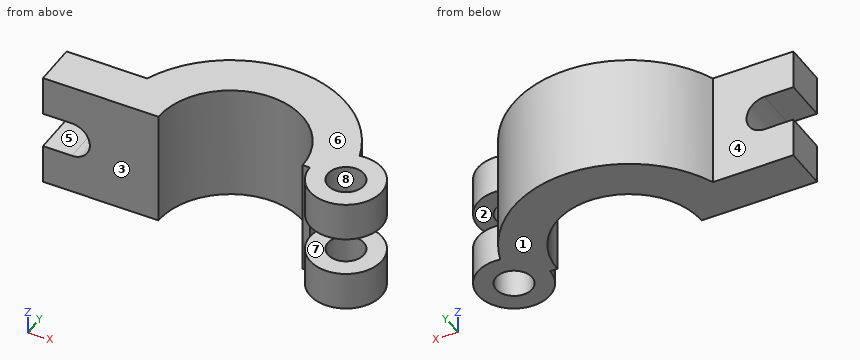
```python
from build123d import *

# Parameters (mm, degrees)
BOSS_EXTRUDE1_DEPTH     = 4
SKETCH2_R               = 2.5
BOSS_EXTRUDE3_DEPTH     = 4
SKETCH3_R               = 1.25
CUT_EXTRUDE1_DEPTH      = 8
SKETCH4_R               = 2.5
CUT_EXTRUDE2_DEPTH      = 1.333333333
CUT_EXTRUDE3_DEPTH      = 15.671400751
CUT_EXTRUDE3_DEPTH_BACK = 3


with BuildPart() as part:
    # Sketch1 → Boss-Extrude1 (new, symmetric)
    with BuildSketch(Plane.XY):
        with BuildLine():
            ThreePointArc((-8, 0), (0, 8), (8, 0))
            Line((8, 0), (5, 0))
            ThreePointArc((5, 0), (0, 5), (-5, 0))
            Line((-5, 0), (-8, 0))
        make_face()
        with BuildLine():
            Line((-13, 0), (-8, 0))
            ThreePointArc((-8, 0), (-7.85269342, 1.5281381), (-7.416198487, 3))
            Line((-7.416198487, 3), (-13, 3))
            Line((-13, 3), (-13, 0))
        make_face()
    extrude(amount=BOSS_EXTRUDE1_DEPTH, both=True)

    # Sketch2 → Boss-Extrude3 (add, symmetric)
    with BuildSketch(Plane.XY):
        with Locations((8, 0)):
            Circle(SKETCH2_R)
    extrude(amount=BOSS_EXTRUDE3_DEPTH, both=True)

    # Sketch3 → Cut-Extrude1 (cut)
    with BuildSketch(Plane.XY.offset(4)):
        with Locations((8, 0)):
            Circle(SKETCH3_R)
    extrude(amount=-CUT_EXTRUDE1_DEPTH, mode=Mode.SUBTRACT)

    # Sketch4 → Cut-Extrude2 (cut, symmetric)
    with BuildSketch(Plane.XY):
        with Locations((8, 0)):
            Circle(SKETCH4_R)
    extrude(amount=CUT_EXTRUDE2_DEPTH, both=True, mode=Mode.SUBTRACT)

    # Sketch5 → Cut-Extrude3 (cut, two sides: drawn at the far end of the back side and taken through both)
    with BuildSketch(Plane(origin=(0, 3, 0), x_dir=(1, 0, 0), z_dir=(0, 1, 0)).offset(-CUT_EXTRUDE3_DEPTH_BACK)):
        with BuildLine():
            Line((-11, 1.25), (-13, 1.25))
            Line((-13, 1.25), (-13, -1.25))
            Line((-13, -1.25), (-11, -1.25))
            ThreePointArc((-11, -1.25), (-9.75, 0), (-11, 1.25))
        make_face()
    extrude(amount=CUT_EXTRUDE3_DEPTH + CUT_EXTRUDE3_DEPTH_BACK, mode=Mode.SUBTRACT)


solid = part.part
```
Part model, mm, in its own coordinate system. Face numbers are marked on the shaded views. A direction names the side the tool comes from. Coordinates: 2 decimals unless noted, no trailing zeros. Order: outer loops, then holes, each group sorted by start corner. A loop starts at its lowest first (then second) coordinate and runs counter-clockwise, first axis right, second up. Notation, with made-up numbers: (-15.75, -8.5) -> (12.25, -8.5) arc R30 cw to (12.25, 26.5) -> close; hole circle Ø1 at (78, -20). An arc over 180 degrees is marked (long way). Put each result on its own line as item: value. Start each with the question number.
(1) Band-saw the part on A-A (z = 3.25). Give the cut face in (x, y).
(2) Band-saw the part on B-B (x = 8). Give the cut face in (y, z).
(3) Band-saw the part on C-C (y = 4.25). Give the cut face in (x, z).
(4) Band-saw the part on D-D (y = 0.5). Give the cut face in (x, z).
(5) Mould opens along Z. For the marked faces 6, 7 and 8 say: pulls with the +Z half, pulls with the -Z half, needs draft (parallel to the pull), parting line crosses it, or undercut.
(6) Pin check, flat tips, straight feed: pin 1 Ø2.5 at (x, y) = (9, 0.5) entering from -Z; pin 2 Ø0.6 at (x, z) = (5, 0.5) entering from -Y; pin 3 Ø1.5 at (x, y) = (8, 0) entering from +Z; pin 4 Ø4.5 at (x, z) = (-11, 1.5) entering from +Y. Stop position of each tip, or through.
(7) Which spindle directions (+Z, -Z, +X, -X, +Y, -Y) get a long thin tool onto all of the face, cutting with end or side? Do the marked faces 1, 2, 3, 4 and 5. Say none if no direction does.
(8) Probe line 1 along Y through (x, z) = (8, 2.55); line 2 along X through (y, z) = (2, -3.5); line 3 along Y through (x, z) = (-7.5, -3.25). List the from-to ranges inside material, lowest first. Write a range as [from, to].
Determined:
1. outline: (-13, 0) -> (-5, 0) arc R5 cw to (5, 0) -> (5.5, 0) arc R2.5 ccw (long way) to (7.61, 2.47) arc R8 ccw to (-7.42, 3) -> (-13, 3) -> close; hole circle Ø2.5 at (8, 0)
2. outline: (-2.5, -4) -> (-1.25, -4) -> (-1.25, -1.33) -> (-2.5, -1.33) -> close; (-2.5, 1.33) -> (-1.25, 1.33) -> (-1.25, 4) -> (-2.5, 4) -> close; (1.25, -4) -> (2.5, -4) -> (2.5, -1.33) -> (1.25, -1.33) -> close; (1.25, 1.33) -> (2.5, 1.33) -> (2.5, 4) -> (1.25, 4) -> close
3. outline: (-6.78, -4) -> (-2.63, -4) -> (-2.63, 4) -> (-6.78, 4) -> close; (2.63, -4) -> (6.78, -4) -> (6.78, 4) -> (2.63, 4) -> close
4. outline: (-13, -4) -> (-4.97, -4) -> (-4.97, 4) -> (-13, 4) -> (-13, 1.25) -> (-11, 1.25) arc R1.25 cw to (-11, -1.25) -> (-13, -1.25) -> close; (4.97, -4) -> (6.85, -4) -> (6.85, -1.33) -> (5.55, -1.33) -> (5.55, 1.33) -> (6.85, 1.33) -> (6.85, 4) -> (4.97, 4) -> close; (9.15, -4) -> (10.45, -4) -> (10.45, -1.33) -> (9.15, -1.33) -> close; (9.15, 1.33) -> (10.45, 1.33) -> (10.45, 4) -> (9.15, 4) -> close
5. face 6: pulls with the +Z half
5. face 7: undercut
5. face 8: needs draft
6. pin 1: stops at z = -4
6. pin 2: stops at y = 0
6. pin 3: passes through
6. pin 4: stops at y = 3
7. face 1: -Z, +X, -X, +Y, -Y
7. face 2: +X, -Y
7. face 3: +Z, -Z, -X, -Y
7. face 4: +Z, -Z, -X, +Y
7. face 5: -X, +Y, -Y
8. line 1: y = [-2.5, -1.25], [1.25, 2.5]
8. line 2: x = [-13, -4.58], [4.58, 9.5]
8. line 3: y = [0, 3]
